Work out the finished part from the listing and answer in its coordinate system (mm). A direction names the side the tool comes from. Round coordinates to 2 decimals unless told otherwise and drop trailing zeros. Order: outer loops, then holes, each group sorted by start corner. A loop starts at its lowest first (then second) coordinate and runs counter-clockwise, first axis right, second up. Notation, with made-up numbers: M 40.25,23 L 57.25,23 A15 ccw 57.25,47 Z; hole C -37.75,4 d2. An arc over 180 degrees is marked long. Answer as a JSON object with one key per item and string values. Group by question number.
from build123d import *

# Parameters (mm, degrees)
SKETCH1_R                = 1.5875
BOSS_EXTRUDE1_DEPTH      = 16.50746
SKETCH2_R                = 1.19126
BOSS_EXTRUDE2_DEPTH      = 0.381
SKETCH3_R                = 1.5875
BOSS_EXTRUDE3_DEPTH      = 1.27
CHAMFER1_SIZE            = 0.381
CHAMFER1_OF_MIRROR1_SIZE = 0.381


with BuildPart() as part:
    # Sketch1 → Boss-Extrude1 (new body, symmetric)
    with BuildSketch(Plane.XY):
        Circle(SKETCH1_R)
    extrude(amount=BOSS_EXTRUDE1_DEPTH, both=True)

    # Sketch2 → Boss-Extrude2 (add)
    with BuildSketch(Plane.XY.offset(16.50746)):
        Circle(SKETCH2_R)
    boss_extrude2 = extrude(amount=BOSS_EXTRUDE2_DEPTH)

    # Sketch3 → Boss-Extrude3 (add)
    with BuildSketch(Plane.XY.offset(16.88846)):
        Circle(SKETCH3_R)
    boss_extrude3 = extrude(amount=BOSS_EXTRUDE3_DEPTH)

    # Chamfer1
    chamfer1_edges = [part.edges().sort_by_distance(p)[0] for p in [
        (-1.5875, 0, 18.15846),
    ]]
    chamfer(chamfer1_edges, length=CHAMFER1_SIZE)

    # Mirror1: Boss-Extrude2, Boss-Extrude3 across plane
    add(boss_extrude2.mirror(Plane.XY))
    add(boss_extrude3.mirror(Plane.XY))

    # Chamfer1 of Mirror1
    chamfer1_of_mirror1_edges = [part.edges().sort_by_distance(p)[0] for p in [
        (-1.5875, 0, -18.15846),
    ]]
    chamfer(chamfer1_of_mirror1_edges, length=CHAMFER1_OF_MIRROR1_SIZE)


solid = part.part
Item 1: Find section A-A (z = -5). Give the vertices of the cut face in (x, y) (1 decimal).
Item 2: The mould has two halves that part along Z. Classify faces 1 (the flat face through (0, 0, -18.158)), 2 (the flat face through (1, 1, -16.888)), 3 (the cylindrical face through (-0.34, -1.55, 0.23)), 4 (the flat face through (0, 0, 18.158)): +Z half, -Z half, draft (parallel to the pull), parting line (faces both ways), or undercut.
Item 3: A tool of negligible diameter and unlimited length cuts with its end or side. For faces 5 (the cylindrical face through (0.64, 1.004, 16.695)), 6 (the cylindrical face through (-0.34, -1.55, 17.33)), from which of +Z, -Z, +X, -X, +Y, -Y can it reach the whole face along a straight path? Write none if from no direction.
Item 4: Consider L1, parallel to Z at x = 1.25, y = -0.1; L2, parallel to X at y = 1.05, z = -0.5; L3, parallel to X at y = 0.1, z = -14. Determine where each line is inside the solid, lowest interval first.
Responses:
{
 "1": {"outline": "C 0,0 d3.2"},
 "2": {"face 1": "-Z half", "face 2": "undercut", "face 3": "draft", "face 4": "+Z half"},
 "3": {"face 5": "none", "face 6": "+Z, -Z"},
 "4": {"L1": "z = -18.11 to -16.89, -16.51 to 16.51, 16.89 to 18.11", "L2": "x = -1.19 to 1.19", "L3": "x = -1.58 to 1.58"}
}
